```python
from build123d import *

# Parameters (mm, degrees)
EXTRUDE_1_DEPTH     = 23
SKETCH_2_R          = 11
EXTRUDE_2_DEPTH     = 2
SKETCH_3_R          = 2.5
EXTRUDE_3_DEPTH     = 23
SKETCH_4_R          = 1.55
CUT_EXTRUDE_1_DEPTH = 5


with BuildPart() as part:
    # 草图1 → 凸台-拉伸1 (new body)
    with BuildSketch(Plane.XY):
        with BuildLine():
            Line((-18, 21), (18, 21))
            ThreePointArc((18, 21), (20.121320344, 20.121320344), (21, 18))
            Line((21, 18), (21, -18))
            ThreePointArc((21, -18), (20.121320344, -20.121320344), (18, -21))
            Line((18, -21), (-18, -21))
            ThreePointArc((-18, -21), (-20.121320344, -20.121320344), (-21, -18))
            Line((-21, -18), (-21, 18))
            ThreePointArc((-21, 18), (-20.121320344, 20.121320344), (-18, 21))
        make_face()
    extrude(amount=EXTRUDE_1_DEPTH)

    # 草图2 → 凸台-拉伸2 (add)
    with BuildSketch(Plane.XY.offset(23)):
        Circle(SKETCH_2_R)
    extrude(amount=EXTRUDE_2_DEPTH)

    # 草图3 → 凸台-拉伸3 (add)
    with BuildSketch(Plane.XY.offset(25)):
        Circle(SKETCH_3_R)
    extrude(amount=EXTRUDE_3_DEPTH)

    # 草图4 → 切除-拉伸1 (cut)
    with BuildSketch(Plane.XY.offset(23)):
        with Locations((-15.5, 15.5)):
            Circle(SKETCH_4_R)
        with Locations((15.5, 15.5)):
            Circle(SKETCH_4_R)
        with Locations((15.5, -15.5)):
            Circle(SKETCH_4_R)
        with Locations((-15.5, -15.5)):
            Circle(SKETCH_4_R)
    extrude(amount=-CUT_EXTRUDE_1_DEPTH, mode=Mode.SUBTRACT)


solid = part.part
```
Design review of the part built by this model. Coordinates are the model's own, in mm. A direction names the side the tool comes from. Give positions to 0.01 mm unless a question says otherwise; leave off trailing zeros. Order: outer loops, then holes, each group sorted by start corner. A loop starts at its lowest first (then second) coordinate and runs counter-clockwise, first axis right, second up. Notation, with made-up numbers: (32.5, 10.5) - (62.5, 10.5) arc R7 ccw to (62.5, 16.5) - close; hole circle Ø2 at (36.25, 3). An arc over 180 degrees is marked (long way). Use a Markdown table: item, result. Add a question column.
(1) Add section B-B on y = -15.5. Give the boundary of the cut face in (x, z).
(2) Add section C-C on z = 37.5. Give the boundary of the cut face in (x, y), then the cut area to 3 significant figures.
(3) Mouldability with a two-part tool opening along Y and no side actions: class faces 3 (the face through (0, 21, 11)), 4 (the face through (15, 16, 18)), 5 (the face through (-0.54, -2.44, 36.34)) as +Y half, -Y half, draft (parallel to the pull), parting line (faces both ways), or undercut.
(4) Clearance check with flat-ended pins moving along their axes: P1, Ø0.9, axis at x = 15.5, y = 15, coming from the +Z side; P2, Ø8, axis at x = 7.5, y = -2, coming from the +Z side; P3, Ø5, axis at x = 15.5, y = -15.5, coming from the +Z side. State where each tip first meets the part, or that it passes through.
(5) Add section A-A on x = 0. Give the boundary of the cut face in (y, z), then the cut area to 4 significant figures.
(6) Machinability: for faces 1 (the face through (0, -21, 11)), 2 (the face through (-16.64, -14.45, 20.54)), which of the approach directions +Z, -Z, +X, -X, +Y, -Y give a long, thin tool a straight path to every point of the face, cutting with its end or side? Answer none if there is none.
(7) Wall thickness on probe 1 along Y at (x, z) = (15.5, 20.6); probe 2 along X at (y, z) = (15, 21); probe 3 along Z at (x, y) = (-17, 1.5): over which ranges is each line inside the solid? List them lowest first. Write a range as [from, to].
(8) Add section D-D on x = 9. Give the boundary of the cut face in (y, z).
Report:
| question | item | result |
|---|---|---|
| 1 | outline | (-21, 0) - (21, 0) - (21, 23) - (17.05, 23) - (17.05, 18) - (13.95, 18) - (13.95, 23) - (-13.95, 23) - (-13.95, 18) - (-17.05, 18) - (-17.05, 23) - (-21, 23) - close |
| 2 | outline | circle Ø5 at (0, 0) |
| 2 | area | 19.6 mm² |
| 3 | face 3 | +Y half |
| 3 | face 4 | undercut |
| 3 | face 5 | parting line |
| 4 | P1 | stops at z = 18 |
| 4 | P2 | stops at z = 25 |
| 4 | P3 | stops at z = 23 |
| 5 | outline | (-21, 0) - (21, 0) - (21, 23) - (11, 23) - (11, 25) - (2.5, 25) - (2.5, 48) - (-2.5, 48) - (-2.5, 25) - (-11, 25) - (-11, 23) - (-21, 23) - close |
| 5 | area | 1,125 mm² |
| 6 | face 1 | +Z, -Z, +X, -X, -Y |
| 6 | face 2 | +Z |
| 7 | probe 1 | y = [-21, -17.05], [-13.95, 13.95], [17.05, 21] |
| 7 | probe 2 | x = [-21, -16.97], [-14.03, 14.03], [16.97, 21] |
| 7 | probe 3 | z = [0, 23] |
| 8 | outline | (-21, 0) - (21, 0) - (21, 23) - (6.32, 23) - (6.32, 25) - (-6.32, 25) - (-6.32, 23) - (-21, 23) - close |
